Here's how the part is built. I have some questions about the finished solid (model axes, mm). Coordinates: 2 decimals unless noted, no trailing zeros. Order: outer loops, then holes, each group sorted by start corner. A loop starts at its lowest first (then second) coordinate and runs counter-clockwise, first axis right, second up. Notation, with made-up numbers: (-8, 72) - (37, 72) arc R32 cw to (37, 99) - close; hole circle Ø1 at (55, 30.5). An arc over 180 degrees is marked (long way). Answer in a Markdown table with one row per item. Add a question column.
Item 1: I want a section at B-B (y = 0.95). Please give me the cut outline in (x, z).
Item 2: Will this pin go through, and if not, where does the flat tip stop? pin 1 Ø1 at (x, y) = (-53, 1.5) entering from +Z.
Item 3: I want a section at A-A (x = -20). Please give me the cut outline in (y, z), plus the area to 3 significant figures.
Item 4: If I drill on line 1 along Z through (x, y) = (-7.5, 0.8); line 2 along X through (y, z) = (0.85, 16); line 3 along Z through (x, y) = (-51, 0.8), over which ranges is the centre line in solid material (lowest first)? Write a range as from..to.
Item 5: I want a section at C-C (z = -0.5). Please give me the cut outline in (x, y), plus the area to 3 significant figures.
Item 6: I want a section at D-D (x = -50). Please give me the cut outline in (y, z).
```python
from build123d import *

# Parameters (mm, degrees)
BOSS_EXTRUDE1_DEPTH = 2


with BuildPart() as part:
    # Sketch1 → Boss-Extrude1 (new body)
    with BuildSketch(Plane(origin=(0, 0, 0), x_dir=(1, 0, 0), z_dir=(0, 1, 0))):
        with BuildLine():
            Line((-39.5, -16), (-39.5, 13))
            Line((-39.5, 13), (-59.5, 13))
            Line((-59.5, 13), (-59.5, -18))
            Line((-59.5, -18), (-64.5, -18))
            Line((-64.5, -18), (-64.5, 18))
            Line((-64.5, 18), (-39.5, 18))
            Line((-39.5, 18), (37.5, 18))
            ThreePointArc((37.5, 18), (38.914213562, 17.414213562), (39.5, 16))
            Line((39.5, 16), (39.5, -16))
            ThreePointArc((39.5, -16), (38.914213562, -17.414213562), (37.5, -18))
            Line((37.5, -18), (-37.5, -18))
            ThreePointArc((-37.5, -18), (-38.914213562, -17.414213562), (-39.5, -16))
        make_face()
        with BuildLine():
            Line((-25, 11), (27.5, 11))
            ThreePointArc((27.5, 11), (28.914213562, 10.414213562), (29.5, 9))
            Line((29.5, 9), (29.5, 6.5))
            ThreePointArc((29.5, 6.5), (28.181980515, 3.318019485), (25, 2))
            Line((25, 2), (-27.5, 2))
            ThreePointArc((-27.5, 2), (-28.914213562, 2.585786438), (-29.5, 4))
            Line((-29.5, 4), (-29.5, 6.5))
            ThreePointArc((-29.5, 6.5), (-28.181980515, 9.681980515), (-25, 11))
        make_face(mode=Mode.SUBTRACT)
        with BuildLine():
            Line((-27.5, -4), (25, -4))
            ThreePointArc((25, -4), (28.181980515, -5.318019485), (29.5, -8.5))
            Line((29.5, -8.5), (29.5, -11))
            ThreePointArc((29.5, -11), (28.914213562, -12.414213562), (27.5, -13))
            Line((27.5, -13), (-25, -13))
            ThreePointArc((-25, -13), (-28.181980515, -11.681980515), (-29.5, -8.5))
            Line((-29.5, -8.5), (-29.5, -6))
            ThreePointArc((-29.5, -6), (-28.914213562, -4.585786438), (-27.5, -4))
        make_face(mode=Mode.SUBTRACT)
    extrude(amount=BOSS_EXTRUDE1_DEPTH)


solid = part.part
```
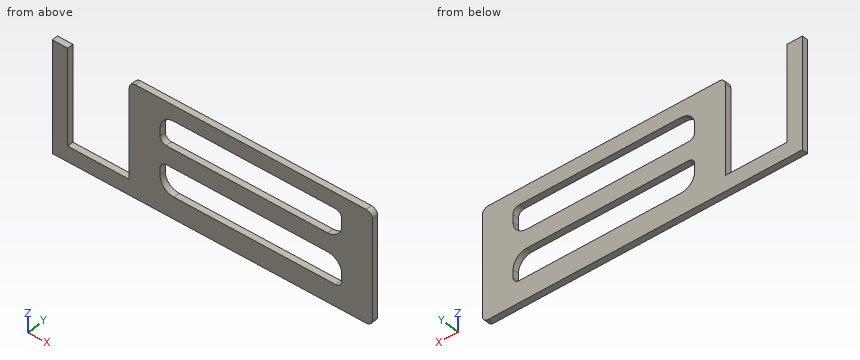
Values follow:
| question | item | result |
|---|---|---|
| 1 | outline | (-64.5, -18) - (37.5, -18) arc R2 ccw to (39.5, -16) - (39.5, 16) arc R2 ccw to (37.5, 18) - (-37.5, 18) arc R2 ccw to (-39.5, 16) - (-39.5, -13) - (-59.5, -13) - (-59.5, 18) - (-64.5, 18) - close; hole (-29.5, -6.5) arc R4.5 ccw to (-25, -11) - (27.5, -11) arc R2 ccw to (29.5, -9) - (29.5, -6.5) arc R4.5 ccw to (25, -2) - (-27.5, -2) arc R2 ccw to (-29.5, -4) - close; hole (-29.5, 6) arc R2 ccw to (-27.5, 4) - (25, 4) arc R4.5 ccw to (29.5, 8.5) - (29.5, 11) arc R2 ccw to (27.5, 13) - (-25, 13) arc R4.5 ccw to (-29.5, 8.5) - close |
| 2 | pin 1 | stops at z = -13 |
| 3 | outline | (0, -18) - (2, -18) - (2, -11) - (0, -11) - close; (0, -2) - (2, -2) - (2, 4) - (0, 4) - close; (0, 13) - (2, 13) - (2, 18) - (0, 18) - close |
| 3 | area | 36.0 mm^2 |
| 4 | line 1 | z = -18..-11, -2..4, 13..18 |
| 4 | line 2 | x = -64.5..-59.5, -39.5..39.5 |
| 4 | line 3 | z = -18..-13 |
| 5 | outline | (-64.5, 0) - (-59.5, 0) - (-59.5, 2) - (-64.5, 2) - close; (-39.5, 0) - (39.5, 0) - (39.5, 2) - (-39.5, 2) - close |
| 5 | area | 168 mm^2 |
| 6 | outline | (0, -18) - (2, -18) - (2, -13) - (0, -13) - close |
